Part model, mm, in its own coordinate system. A direction names the side the tool comes from. Give positions to 0.01 mm unless a question says otherwise; leave off trailing zeros. Order: outer loops, then holes, each group sorted by start corner. A loop starts at its lowest first (then second) coordinate and runs counter-clockwise, first axis right, second up. Notation, with made-up numbers: M -17,39 L -10,39 A27 ccw -10,60 Z; hole C -18.75,85.5 d4. An arc over 180 degrees is marked long. Answer as a JSON object with one key per item and string values.
from build123d import *

# Parameters (mm, degrees)
SKETCH1_R           = 4
BOSS_EXTRUDE1_DEPTH = 8


with BuildPart() as part:
    # Sketch1 → Boss-Extrude1 (new body)
    with BuildSketch(Plane(origin=(0, 0, 0), x_dir=(0, 1, 0), z_dir=(0, 0, 1))):
        with BuildLine():
            ThreePointArc((16.820508076, 10.866025404), (14.05137554, 10.65443031), (11.444646973, 9.696393951))
            ThreePointArc((11.444646973, 9.696393951), (10.606601718, 10.606601718), (9.696393951, 11.444646973))
            ThreePointArc((9.696393951, 11.444646973), (10.668335485, 14.048350177), (10.866025404, 16.820508076))
            Line((10.866025404, 16.820508076), (9.133974596, 17.820508076))
            ThreePointArc((9.133974596, 17.820508076), (6.841633021, 16.252695081), (5.063158041, 14.119646973))
            ThreePointArc((5.063158041, 14.119646973), (3.882285677, 14.488887394), (2.675, 14.759551992))
            ThreePointArc((2.675, 14.759551992), (2.214874458, 17.500395877), (1, 20))
            Line((1, 20), (-1, 20))
            ThreePointArc((-1, 20), (-2.201319541, 17.496063331), (-2.675, 14.759551992))
            ThreePointArc((-2.675, 14.759551992), (-3.882285677, 14.488887394), (-5.063158041, 14.119646973))
            ThreePointArc((-5.063158041, 14.119646973), (-6.832060392, 16.263224635), (-9.133974596, 17.820508076))
            Line((-9.133974596, 17.820508076), (-10.866025404, 16.820508076))
            ThreePointArc((-10.866025404, 16.820508076), (-10.65443031, 14.05137554), (-9.696393951, 11.444646973))
            ThreePointArc((-9.696393951, 11.444646973), (-10.606601718, 10.606601718), (-11.444646973, 9.696393951))
            ThreePointArc((-11.444646973, 9.696393951), (-14.048350177, 10.668335485), (-16.820508076, 10.866025404))
            Line((-16.820508076, 10.866025404), (-17.820508076, 9.133974596))
            ThreePointArc((-17.820508076, 9.133974596), (-16.252695081, 6.841633021), (-14.119646973, 5.063158041))
            ThreePointArc((-14.119646973, 5.063158041), (-14.488887394, 3.882285677), (-14.759551992, 2.675))
            ThreePointArc((-14.759551992, 2.675), (-17.500395877, 2.214874458), (-20, 1))
            Line((-20, 1), (-20, -1))
            ThreePointArc((-20, -1), (-17.496063331, -2.201319541), (-14.759551992, -2.675))
            ThreePointArc((-14.759551992, -2.675), (-14.488887394, -3.882285677), (-14.119646973, -5.063158041))
            ThreePointArc((-14.119646973, -5.063158041), (-16.263224635, -6.832060392), (-17.820508076, -9.133974596))
            Line((-17.820508076, -9.133974596), (-16.820508076, -10.866025404))
            ThreePointArc((-16.820508076, -10.866025404), (-14.05137554, -10.65443031), (-11.444646973, -9.696393951))
            ThreePointArc((-11.444646973, -9.696393951), (-10.606601718, -10.606601718), (-9.696393951, -11.444646973))
            ThreePointArc((-9.696393951, -11.444646973), (-10.668335485, -14.048350177), (-10.866025404, -16.820508076))
            Line((-10.866025404, -16.820508076), (-9.133974596, -17.820508076))
            ThreePointArc((-9.133974596, -17.820508076), (-6.841633021, -16.252695081), (-5.063158041, -14.119646973))
            ThreePointArc((-5.063158041, -14.119646973), (-3.882285677, -14.488887394), (-2.675, -14.759551992))
            ThreePointArc((-2.675, -14.759551992), (-2.214874458, -17.500395877), (-1, -20))
            Line((-1, -20), (1, -20))
            ThreePointArc((1, -20), (2.201319541, -17.496063331), (2.675, -14.759551992))
            ThreePointArc((2.675, -14.759551992), (3.882285677, -14.488887394), (5.063158041, -14.119646973))
            ThreePointArc((5.063158041, -14.119646973), (6.832060392, -16.263224635), (9.133974596, -17.820508076))
            Line((9.133974596, -17.820508076), (10.866025404, -16.820508076))
            ThreePointArc((10.866025404, -16.820508076), (10.65443031, -14.05137554), (9.696393951, -11.444646973))
            ThreePointArc((9.696393951, -11.444646973), (10.606601718, -10.606601718), (11.444646973, -9.696393951))
            ThreePointArc((11.444646973, -9.696393951), (14.048350177, -10.668335485), (16.820508076, -10.866025404))
            Line((16.820508076, -10.866025404), (17.820508076, -9.133974596))
            ThreePointArc((17.820508076, -9.133974596), (16.252695081, -6.841633021), (14.119646973, -5.063158041))
            ThreePointArc((14.119646973, -5.063158041), (14.488887394, -3.882285677), (14.759551992, -2.675))
            ThreePointArc((14.759551992, -2.675), (17.500395877, -2.214874458), (20, -1))
            Line((20, -1), (20, 1))
            ThreePointArc((20, 1), (17.496063331, 2.201319541), (14.759551992, 2.675))
            ThreePointArc((14.759551992, 2.675), (14.488887394, 3.882285677), (14.119646973, 5.063158041))
            ThreePointArc((14.119646973, 5.063158041), (16.263224635, 6.832060392), (17.820508076, 9.133974596))
            Line((17.820508076, 9.133974596), (16.820508076, 10.866025404))
        make_face()
        with Locations(Location((0, 0, 0), (0, 0, 270))):
            Circle(SKETCH1_R, mode=Mode.SUBTRACT)
    extrude(amount=BOSS_EXTRUDE1_DEPTH)


solid = part.part
1. Cut at C-C on x = -16. Give the cut face in (y, z), plus the area to 3 significant figures.
Worked answers:
{"outline": "M -10.88,0 L -6.55,0 L -6.55,8 L -10.88,8 Z; M -2.56,0 L 2.57,0 L 2.57,8 L -2.56,8 Z; M 6.57,0 L 10.89,0 L 10.89,8 L 6.57,8 Z", "area": "110 mm^2"}
2. Cut at D-D on y = 8. Give the cut face in (x, z).
Worked answers:
{"outline": "M -17.16,0 L 17.17,0 L 17.17,8 L -17.16,8 Z"}
3. Cut at A-A on y = 0. Give the cut face in (x, z).
Worked answers:
{"outline": "M -20,0 L -4,0 L -4,8 L -20,8 Z; M 4,0 L 20,0 L 20,8 L 4,8 Z"}
4. Two-plate mould, pull along Y, no slides. Class faces 1 (the cylindrical face through (-14.493, -3.866, 3.944)), 2 (the cylindrical face through (3.899, 14.484, 3.944)), 3 (the flat face through (4.2, -0.3, 8)): +Y half, -Y half, draft (parallel to the pull), parting line (faces both ways), or undercut.
Worked answers:
{"face 1": "undercut", "face 2": "+Y half", "face 3": "draft"}
5. Which spindle directions (+Z, -Z, +X, -X, +Y, -Y) get a long thin tool onto all of the face, cutting with end or side? Do faces 4 (the cylindrical face through (-2.227, -17.463, 3.944)), 5 (the flat face through (4.2, -0.3, 0)), 6 (the cylindrical face through (16.237, 6.803, 3.944)), 7 (the cylindrical face through (-16.28, 6.87, 3.94)), 8 (the cylindrical face through (10.594, -10.619, 3.944)). Say none if no direction does.
Worked answers:
{"face 4": "+Z, -Z, -Y", "face 5": "-Z, +X, -X, +Y, -Y", "face 6": "+Z, -Z, +X", "face 7": "+Z, -Z, -X", "face 8": "+Z, -Z"}
6. Pin check, flat tips, straight feed: P1, Ø3, axis at y = 5.5, z = 1.5, coming from the -X side; P2, Ø4, axis at y = -11.5, z = 1, coming from the -X side. Stop position of each tip, or through.
Worked answers:
{"P1": "stops at x = -16.39", "P2": "stops at x = -17.61"}
7. Probe line 1 along Y through (x, z) = (-16, 3.25); line 2 along Y through (x, z) = (0, 3.5); line 3 along X through (y, z) = (-17, 5.25). List the from-to ranges inside material, lowest first.
Worked answers:
{"line 1": "y = -10.88 to -6.55, -2.56 to 2.57, 6.57 to 10.89", "line 2": "y = -20 to -4, 4 to 20", "line 3": "x = -10.56 to -7.77, -2.36 to 2.35, 7.75 to 10.56"}
